Here's how the part is built. I have some questions about the finished solid (model axes, mm). A direction names the side the tool comes from. Coordinates: 2 decimals unless noted, no trailing zeros. Loops run counter-clockwise (first coordinate to the right, second up) from the corner with the lowest first, then second, coordinate; pieces in that order, holes last. Notation, with made-up numbers: M 74.5,58.25 L 110.5,58.25 A35 cw 110.5,91.25 Z; hole C -0.75,-37 d4. An arc over 180 degrees is marked long. Use CSV: the item, a comma, the result in double quotes. Start each with the question number.
Q1. If we section it at C-C (y = -17): Please give me the cut outline in (x, z), and give its area (3 significant figures).
Q2. Which directions (+Z, -Z, +X, -X, +Y, -Y) give clear straight access to the entire face, cutting with the end or side of a thin tool? Please do faces 4 (the cylindrical face through (-19.946, -23.846, -7.509)), 5 (the flat face through (139.774, 0, 0)), 6 (the cylindrical face through (49.91, 19.98, -0.88)).
Q3. If we section it at A-A (z = -13): Please give me the cut outline in (x, y), and give its area (3 significant figures).
Q4. If we mould it in two halves opening along Z, with no side actions, what happens to faces 1 (the flat face through (119.774, -2, 2)), 2 (the cylindrical face through (129.9, 2.5, -0.1)), 3 (the flat face through (-0.123, 0, 0))? For each: +Z half, -Z half, draft (parallel to the pull), parting line (faces both ways), or undercut.
Q5. For pin 1 Ø12 at (y, z) = (-2.5, 1.5) entering from +X; pin 2 Ø24 at (y, z) = (1, 5) entering from -X; pin 3 Ø10 at (x, y) = (42, 16.5) entering from -Z; pin 4 Ø3 at (x, y) = (59.5, 2.5) entering from +Z (3 decimals), each with a flat end and sliding along its axis, tell me the tip position at first contact or that it passes through.
Q6. If we section it at B-B (x = -7): Please give me the cut outline in (y, z).
Q7. If we section it at D-D (x = 86): Please give me the cut outline in (y, z).
Q8. Please list where these lines run through material, in increasing order: probe 1 along Z at (x, y) = (-19, 0); probe 2 along X at (y, z) = (6, 34.5); probe 3 along X at (y, z) = (-10.5, -18.5). Write a range as [from, to].
from build123d import *


with BuildPart() as part:
    # Sketch1 → Revolve2 (revolve)
    with BuildSketch(Plane.XY, mode=Mode.PRIVATE) as revolve2_sk:
        Polygon((-40.225741407, 20), (-40.225741407, 25), (-0.225741407, 25), (-0.225741407, 40), (19.774258593, 40), (19.774258593, 25), (39.774258593, 25), (39.774258593, 20), (59.774258593, 20), (59.774258593, 15), (79.774258593, 15), (79.774258593, 10), (99.774258593, 10), (99.774258593, 5), (119.774258593, 5), (119.774258593, 2.5), (139.774258593, 2.5), (139.774258593, 0), (-0.122966015, 0), (-0.122966015, 20), align=None)
    revolve(revolve2_sk.sketch.rotate(Axis((-74.790093539, 0, 0), (1, 0, 0)), 180), axis=Axis((-74.790093539, 0, 0), (1, 0, 0)))  # turned: the seam where the file's is


solid = part.part
Results below:
1,outline,"M -40.23,-18.33 L -0.23,-18.33 L -0.23,-36.21 L 19.77,-36.21 L 19.77,-18.33 L 39.77,-18.33 L 39.77,-10.54 L 59.77,-10.54 L 59.77,10.54 L 39.77,10.54 L 39.77,18.33 L 19.77,18.33 L 19.77,36.21 L -0.23,36.21 L -0.23,18.33 L -40.23,18.33 L -40.23,10.54 L -0.12,10.54 L -0.12,-10.54 L -40.23,-10.54 Z"
1,area,"3,220 mm^2"
2,face 4,"-X"
2,face 5,"+Z, -Z, +X, +Y, -Y"
2,face 6,"+X"
3,outline,"M -40.23,-21.35 L -0.23,-21.35 L -0.23,-37.83 L 19.77,-37.83 L 19.77,-21.35 L 39.77,-21.35 L 39.77,-15.2 L 59.77,-15.2 L 59.77,-7.48 L 79.77,-7.48 L 79.77,7.48 L 59.77,7.48 L 59.77,15.2 L 39.77,15.2 L 39.77,21.35 L 19.77,21.35 L 19.77,37.83 L -0.23,37.83 L -0.23,21.35 L -40.23,21.35 L -40.23,15.2 L -0.12,15.2 L -0.12,-15.2 L -40.23,-15.2 Z"
3,area,"3,760 mm^2"
4,face 1,"draft"
4,face 2,"parting line"
4,face 3,"undercut"
5,pin 1,"x = 139.77"
5,pin 2,"x = -0.12"
5,pin 3,"z = -21.92"
5,pin 4,"z = 19.975"
6,outline,"C 0,0 d50; hole C 0,0 d40"
7,outline,"C 0,0 d20"
8,probe 1,"[-25, -20], [20, 25]"
8,probe 2,"[-0.23, 19.77]"
8,probe 3,"[-40.23, 39.77]"
